Design review of the part shown in the three views and the two pictorial views. Dimensions are in mm from the part's minimum x, y and z. Give positions to 0.01 mm unless a question says otherwise; leave off trailing zeros. Loops run counter-clockwise (first coordinate to the right, second up) from the corner with the lowest first, then second, coordinate; pieces in that order, holes last.
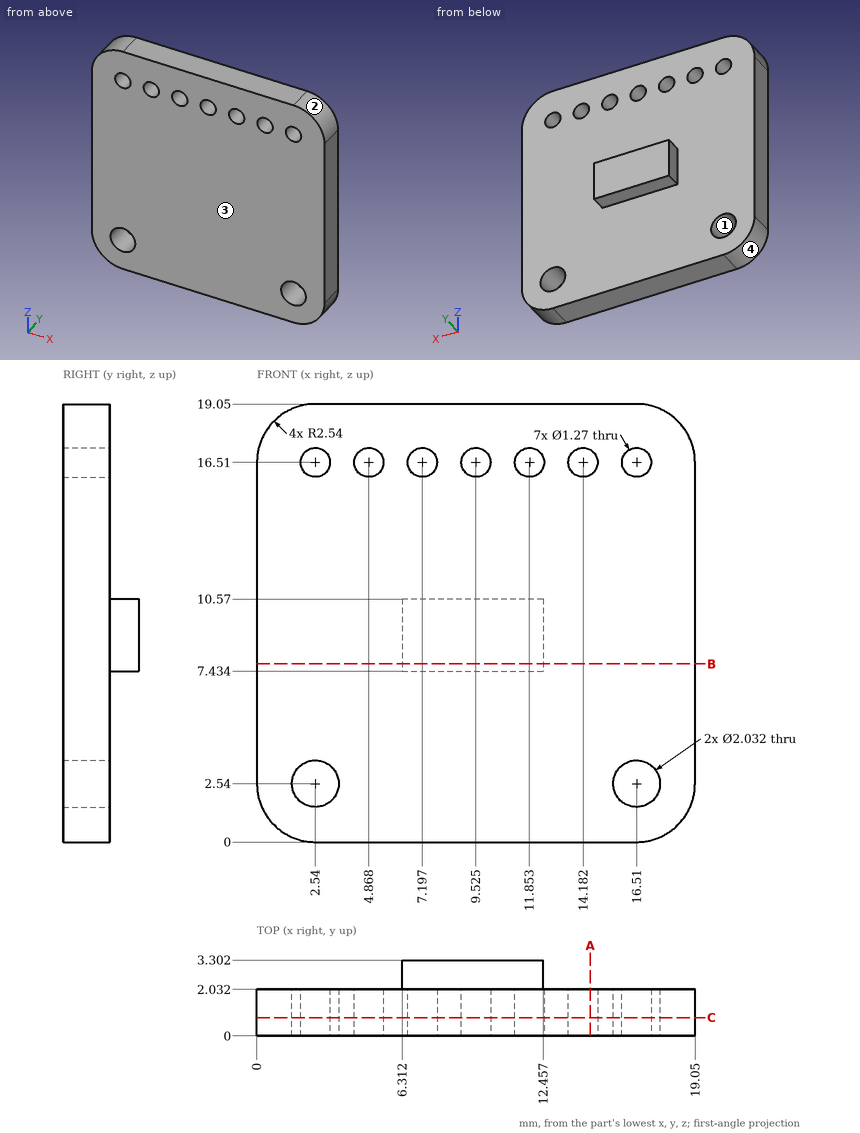
Q1. Consider section A-A on x = 14.5. Give the boundary of the cut face in (y, z).
Answers:
outline: (0, 0) - (2.03, 0) - (2.03, 15.96) - (0, 15.96) - close; (0, 17.06) - (2.03, 17.06) - (2.03, 19.05) - (0, 19.05) - close
Q2. For probe 1 along X at (y, z) = (1.4, 2.54); probe 2 along Z at (x, y) = (16.25, 1.9); probe 3 along Y at (x, z) = (13, 4.25), list the stretches that pass through material, from the lowest coordinate up.
Answers:
probe 1: x = 0 to 1.52, 3.56 to 15.49, 17.53 to 19.05
probe 2: z = 0 to 1.56, 3.52 to 15.93, 17.09 to 19.05
probe 3: y = 0 to 2.03
Q3. Consider section B-B on z = 7.75. Give the boundary of the cut face in (x, y).
Answers:
outline: (0, 0) - (19.05, 0) - (19.05, 2.03) - (12.46, 2.03) - (12.46, 3.3) - (6.31, 3.3) - (6.31, 2.03) - (0, 2.03) - close
Q4. For pin 1 Ø0.8 at (x, z) = (7.2, 16.51) entering from +Y; pin 2 Ø2.5 at (x, z) = (16.51, 2.54) entering from +Y; pin 3 Ø0.6 at (x, y) = (8, 2.5) entering from +Z, all flat-tipped, find the tip position at first contact; note any pin that passes through.
Answers:
pin 1: passes through
pin 2: stops at y = 2.03
pin 3: stops at z = 10.57
Q5. Consider section C-C on y = 0.8. Count the separate pieces of the cut face and the enclosed holes in it, plus the area to 3 significant figures.
Answers:
separate pieces: 1
enclosed holes: 9
area: 342 mm2
Q6. Mouldability with a two-part tool opening along X and no side actions: class the marked faces 1, 2, 3 and 4 as +X half, -X half, draft (parallel to the pull), parting line (faces both ways), or undercut.
Answers:
face 1: undercut
face 2: +X half
face 3: draft
face 4: -X half
